Can you work these out from the model? Positions are in its coordinate system, mm. A direction names the side the tool comes from. Give positions to 0.01 mm unless a question says otherwise; leave off trailing zeros. Order: outer loops, then holes, each group sorted by start corner. A loop starts at its lowest first (then second) coordinate and runs counter-clockwise, first axis right, second up. Notation, with made-up numbers: M 1,30 L 42,30 A29 cw 42,53 Z; hole C 40.25,-12 d2. An arc over 180 degrees is marked long. Write each question's results on one line, items separated by ' | '.
from build123d import *

# Parameters (mm, degrees)
BOSS_EXTRUDE1_DEPTH = 30
SKETCH3_R           = 6.5
SKETCH3_R_2         = 3.75
BOSS_EXTRUDE2_DEPTH = 20
SKETCH4_W           = 3.872983346
SKETCH4_H           = 3
CUT_EXTRUDE1_DEPTH  = 20
FILLET1_R           = 1


with BuildPart() as part:
    # Sketch1 → Boss-Extrude1 (new body)
    with BuildSketch(Plane.XY):
        Polygon((-25, -1.5), (25, -1.5), (25, 1.5), (25, 7.5), (23, 7.5), (23, 1.5), (16, 1.5), (16, 7.5), (14, 7.5), (14, 1.5), (-21.127016654, 1.5), align=None)
    extrude(amount=BOSS_EXTRUDE1_DEPTH)

    # Sketch3 → Boss-Extrude2 (add)
    with BuildSketch(Plane.XY.offset(30)):
        with Locations((-25, 5)):
            Circle(SKETCH3_R)
        with Locations((-25, 5)):
            Circle(SKETCH3_R_2, mode=Mode.SUBTRACT)
    extrude(amount=-BOSS_EXTRUDE2_DEPTH)

    # Sketch4 → Cut-Extrude1 (cut)
    with BuildSketch(Plane(origin=(0, 0, 10), x_dir=(-1, 0, 0), z_dir=(0, 0, -1))):
        with Locations((23.063508327, 0)):
            Rectangle(SKETCH4_W, SKETCH4_H)
    extrude(amount=CUT_EXTRUDE1_DEPTH, mode=Mode.SUBTRACT)

    # Fillet1
    fillet1_edges = [part.edges().sort_by_distance(p)[0] for p in [
        (16, 7.5, 15),
        (23, 7.5, 15),
        (-21.127016654, 1.5, 5),
    ]]
    fillet(fillet1_edges, radius=FILLET1_R)


solid = part.part
(1) Imagine slicing it at D-D, the plane z = 11.75. Write out the boundary of the cut face in (x, y), plus the area to 3 significant figures.
Data:
outline: M -25,-1.5 L 25,-1.5 L 25,7.5 L 24,7.5 A1 ccw 23,6.5 L 23,1.5 L 16,1.5 L 16,6.5 A1 ccw 15,7.5 L 14,7.5 L 14,1.5 L -19.52,1.5 A6.5 ccw long Z; hole C -25,5 d7.5 | area: 251 mm2
(2) Imagine slicing it at B-B, the plane y = 5. Write out the boundary of the cut face in (x, z).
Data:
outline: M -31.5,10 L -28.75,10 L -28.75,30 L -31.5,30 Z; M -21.25,10 L -18.5,10 L -18.5,30 L -21.25,30 Z; M 14,0 L 16,0 L 16,30 L 14,30 Z; M 23,0 L 25,0 L 25,30 L 23,30 Z
(3) Imagine slicing it at C-C, the plane z = 8.75. Write out the boundary of the cut face in (x, y), plus the area to 3 significant figures.
Data:
outline: M -21.13,-1.5 L 25,-1.5 L 25,7.5 L 24,7.5 A1 ccw 23,6.5 L 23,1.5 L 16,1.5 L 16,6.5 A1 ccw 15,7.5 L 14,7.5 L 14,1.5 L -20.13,1.5 A1 ccw -21.13,0.5 Z | area: 162 mm2
(4) For faces 4 (the face through (-22, 2, 10)), 5 (the face through (23.301, 7.215, 15.21)), 6 (the face through (0, -1.5, 15)), 7 (the face through (14.5, 7.5, 14.8)), which set-ups out of +Z, -Z, +X, -X, +Y, -Y let a thin tool reach every point of the face, with its end or its side?
Data:
face 4: -Z, -X, +Y | face 5: +Z, -Z, +Y | face 6: +Z, -Z, +X, -X, -Y | face 7: +Z, -Z, +X, +Y
(5) We'd pull the mould along X, two halves only. Please class faces 1 (the face through (-21.127, -1, 5)), 2 (the face through (25, 3, 15)), 3 (the face through (23, 4, 15)): +X half, -X half, draft (parallel to the pull), parting line (faces both ways), or undercut.
Data:
face 1: -X half | face 2: +X half | face 3: undercut
(6) Imagine slicing it at A-A, the plane x = -26. Write out the boundary of the cut face in (y, z).
Data:
outline: M -1.42,10 L 1.39,10 L 1.39,30 L -1.42,30 Z; M 8.61,10 L 11.42,10 L 11.42,30 L 8.61,30 Z
(7) I need wall thicknesses on L1, parallel to X at y = 4.75, z = 10.5; L2, parallel to Y at x = -25, z = 23.5; L3, parallel to X at y = 7, z = 20.5. Which ranges of each line are inside material? Lowest first, please. Write a range as from..to.
Data:
L1: x = -31.5..-28.74, -21.26..-18.5, 14..16, 23..25 | L2: y = -1.5..1.25, 8.75..11.5 | L3: x = -31.18..-28.17, -21.83..-18.82, 14..15.87, 23.13..25
(8) Will these pins go through, and if not, where does the flat tip stop? P1, Ø9, axis at x = -10.5, z = 9.5, coming from the +Y side; P2, Ø7, axis at x = -25, y = 5, coming from the -Z side; P3, Ø2, axis at y = -0.5, z = 6, coming from the -X side; P4, Ø7.5, axis at x = 19, z = 8, coming from the +Y side.
Data:
P1: stops at y = 1.5 | P2: passes through | P3: stops at x = -21.13 | P4: stops at y = 7.47
